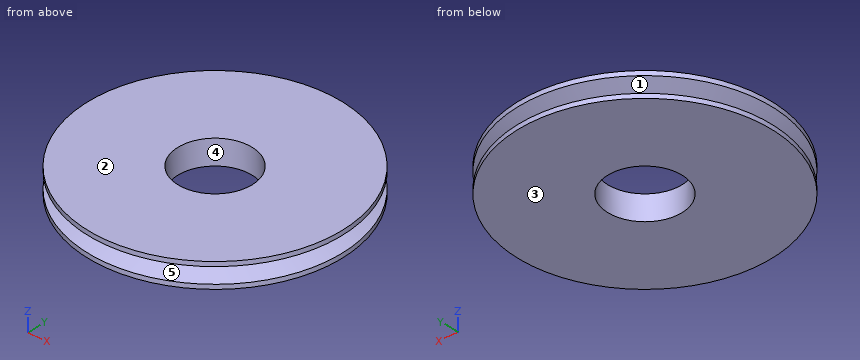
Autodesk Inventor part; units mm, degrees
ref_plane "Plano de correa" through (0, 89, 10) normal (0, 0, 1) x (1, 0, 0)
ref_plane "YZ Plane" through (0, 0, 0) normal (1, 0, 0) x (0, 1, 0)
ref_plane "XZ Plane" through (0, 0, 0) normal (0, 1, 0) x (-1, 0, 0)
sketch "Boceto principal" plane through (0, 0, 0) normal (1, 0, 0) x (0, 1, 0)
  line L0 (0, 20) -> (102.8, 20)
  line L1 (102.8, 20) -> (102.8, 16.356)
  line L2 (102.8, 16.356) -> (89, 12.137)
  line L3 (89, 12.137) -> (89, 7.863)
  line L4 (89, 7.863) -> (102.8, 3.644)
  line L5 (102.8, 3.644) -> (102.8, 0)
  line L6 (102.8, 0) -> (0, 0)
  line L7 (100, 15.5) -> (100, 4.5) construction
  line L8 (89, 10) -> (100, 10) construction
  line L9 (102.8, 16.356) -> (102.8, 3.644)
  line L10 (0, -4) -> (0, 24)
  line L11 (0, 0) -> (0, 20)
  dimension "d0" = 11
  dimension "d1" = 34
  dimension "d2" = 2.8
  dimension "d6" = 20
  dimension "d21" = 200
  dimension "d25" = 13.8
  dimension "d27" = 10
ref_plane "Plano de correa" through (0, 89, 10) normal (0, 0, 1) x (1, 0, 0)
revolve "Cuerpo" add sketch "Boceto principal" angle 360 about axis through (0, 0, -10) along (0, 0, 1)
revolve "Para ranuras" cut sketch "Boceto principal" angle 360 about axis through (0, 0, -10) along (0, 0, 1) contours L9 L4 L3 L2
fillet "Empalme externo" [suppressed]
fillet "Empalme interno" [suppressed]
pattern_of_one "Patrón para ranuras"
sketch "Boceto2" plane through (0, 0, 20) normal (0, 0, 1) x (1, 0, 0)
  circle A0 centre (0, 0) radius 30
  dimension "d28" = 60
extrude "Extrusión1" cut sketch "Boceto2" against normal blind 30
equation "\"d0\" = da_Bw"
equation "\"d1\" = da_Alfa"
equation "\"d2\" = da_c"
equation "\"d21\" = da_Dw"
equation "\"d25\" = da_Hd"
equation "\"d27\" = da_Se"
equation "\"da_r1\" = 0"
equation "\"da_r2\" = 0"
equation "\"d18\" = da_Sg"
equation "\"da_Bw\" = 11"
equation "\"da_Alfa\" = 34deg"
equation "\"da_c\" = 2.8"
equation "\"da_Dw\" = 200"
equation "\"da_Hd\" = 13.8"
equation "\"da_Se\" = 10"
equation "\"da_Sg\" = 15"
properties part number "Polea ranurada2" material "Steel"
Can you work these out from the model? Positions are in its coordinate system, mm. Face numbers are marked on the shaded views. A direction names the side the tool comes from. Give positions to 0.01 mm unless a question says otherwise; leave off trailing zeros. Order: outer loops, then holes, each group sorted by start corner. A loop starts at its lowest first (then second) coordinate and runs counter-clockwise, first axis right, second up. Notation, with made-up numbers: M 48.5,63 L 67.5,63 A22 ccw 67.5,70 Z; hole C 18.25,-33 d7. An arc over 180 degrees is marked long. Use one line per item in the form item = value.
Item 1: Will these pins go through, and if not, where does the flat tip stop? pin 1 Ø12 at (x, z) = (-66, 7.5) entering from +Y; pin 2 Ø12 at (x, z) = (27, 5) entering from +Y; pin 3 Ø10 at (y, z) = (-71, 3) entering from -X.
Values follow:
pin_1 = 82.45
pin_2 = 100.6
pin_3 = -78.82
Item 2: If I drill on line 1 along Y through (x, z) = (0, 11.25); line 2 along Z through (x, y) = (-81.5, -46.5); line 3 along Y through (x, z) = (-8, 11), over which ranges is the centre line in solid material (lowest first)? Write a range as [from, to].
Values follow:
line_1 = [-89, -30], [30, 89]
line_2 = [0, 6.39], [13.61, 20]
line_3 = [-88.64, -28.91], [28.91, 88.64]
Item 3: For the marked faces 4 and 5, which set-ups out of +Z, -Z, +X, -X, +Y, -Y let a thin tool reach every point of the face, with its end or its side?
Values follow:
face_4 = +Z, -Z
face_5 = none
Item 4: Thinking about a two-plate mould opening in Z: for the marked faces 1, 2 and 3, which applies, pulls with the +Z half, pulls with the -Z half, needs draft (parallel to the pull), parting line crosses it, or undercut?
Values follow:
face_1 = undercut
face_2 = pulls with the +Z half
face_3 = pulls with the -Z half
Item 5: If we section it at A-A, the plane y = 0: Write out the boundary of the cut face in (x, z), and give its area (3 significant figures).
Values follow:
outline = M -102.8,0 L -30,0 L -30,20 L -102.8,20 L -102.8,16.36 L -89,12.14 L -89,7.86 L -102.8,3.64 Z; M 30,0 L 102.8,0 L 102.8,3.64 L 89,7.86 L 89,12.14 L 102.8,16.36 L 102.8,20 L 30,20 Z
area = 2,680 mm^2
